CAD build for the part. Positions are in the model's coordinates, mm. A direction names the side the tool comes from. Coordinates: 2 decimals unless noted, no trailing zeros. Order: outer loops, then holes, each group sorted by start corner. A loop starts at its lowest first (then second) coordinate and runs counter-clockwise, first axis right, second up. Notation, with made-up numbers: (78, -15) - (119, -15) arc R12 ccw to (119, 6) - close; hole circle Ø4 at (34, -37). An arc over 180 degrees is marked (long way). Return JSON: item names as keys, results as strings.
from build123d import *


with BuildPart() as f1:
    # F0 (on Right) → F1 (revolve)
    with BuildSketch(Plane.YZ):
        with BuildLine():
            Line((-12.7, 15.875), (-12.7, 16.594964))
            Line((-12.7, 16.594964), (-1.207143, 19.037846))
            ThreePointArc((-1.207143, 19.037846), (-0.33963, 19.569458), (0, 20.528543))
            Line((0, 20.528543), (0, 37.338))
            ThreePointArc((0, 37.338), (-0.223185, 37.876815), (-0.762, 38.1))
            Line((-0.762, 38.1), (-37.338, 38.1))
            ThreePointArc((-37.338, 38.1), (-37.876815, 37.876815), (-38.1, 37.338))
            Line((-38.1, 37.338), (-38.1, 0))
            Line((-38.1, 0), (-19.05, 0))
            Line((-19.05, 0), (-19.05, 15.875))
            Line((-19.05, 15.875), (-12.7, 15.875))
        make_face()
    revolve(axis=Axis((0, -28.575, 0), (0, 1, 0)))


solid = f1.part
Item 1: Band-saw the part on C-C, the plane y = -5.5. List the corners of the cut face in (x, z).
Findings below:
{"outline": "circle Ø76.2 at (0, 0); hole circle Ø36.25 at (0, 0)"}
Item 2: Band-saw the part on B-B, the plane x = 0. List the corners of the cut face in (y, z) (3 decimals), then the cut area to 3 significant figures.
Findings below:
{"outline": "(-38.1, -37.338) arc R0.762 ccw to (-37.338, -38.1) - (-0.762, -38.1) arc R0.762 ccw to (0, -37.338) - (0, -20.529) arc R1.524 ccw to (-1.207, -19.038) - (-12.7, -16.595) - (-12.7, -15.875) - (-19.05, -15.875) - (-19.05, 15.875) - (-12.7, 15.875) - (-12.7, 16.595) - (-1.207, 19.038) arc R1.524 ccw to (0, 20.529) - (0, 37.338) arc R0.762 ccw to (-0.762, 38.1) - (-37.338, 38.1) arc R0.762 ccw to (-38.1, 37.338) - close", "area": "2,240 mm²"}
Item 3: Mould opens along X. For faces 3 (the cylindrical face through (-23.183, -19.306, -30.235)), 4 (the flat face through (-15, -12.7, -6)), 5 (the flat face through (-16, 0, -16)), 6 (the cylindrical face through (-15.497, -15.831, -3.441)) say: released by +X, released by -X, zero draft, split by the parting line, or undercut.
Findings below:
{"face 3": "split by the parting line", "face 4": "undercut", "face 5": "zero draft", "face 6": "undercut"}
Item 4: Wall check: L1, parallel to X at y = -17.25, z = 0 (3 decimals); L2, parallel to Z at x = 33, y = -34; L3, parallel to Y at x = 4, z = 11. Give the ranges that are in metal, low to high. Write a range as [from, to].
Findings below:
{"L1": "x = [-38.1, -15.875], [15.875, 38.1]", "L2": "z = [-19.04, 19.04]", "L3": "y = [-38.1, -19.05]"}
Item 5: Band-saw the part on D-D, the plane y = -24. List the corners of the cut face in (x, z).
Findings below:
{"outline": "circle Ø76.2 at (0, 0)"}
Item 6: Band-saw the part on A-A, the plane z = 0. List the corners of the cut face in (x, y) (3 decimals).
Findings below:
{"outline": "(-38.1, -37.338) arc R0.762 ccw to (-37.338, -38.1) - (37.338, -38.1) arc R0.762 ccw to (38.1, -37.338) - (38.1, -0.762) arc R0.762 ccw to (37.338, 0) - (20.529, 0) arc R1.524 ccw to (19.038, -1.207) - (16.595, -12.7) - (15.875, -12.7) - (15.875, -19.05) - (-15.875, -19.05) - (-15.875, -12.7) - (-16.595, -12.7) - (-19.038, -1.207) arc R1.524 ccw to (-20.529, 0) - (-37.338, 0) arc R0.762 ccw to (-38.1, -0.762) - close"}
Item 7: Which spindle directions (+Z, -Z, +X, -X, +Y, -Y) get a long thin tool onto all of the face, cutting with end or side? Do faces 1 (the flat face through (0, -19.05, 0)), 2 (the flat face through (1, -38.1, -1)). Say none if no direction does.
Findings below:
{"face 1": "+Y", "face 2": "+Z, -Z, +X, -X, -Y"}
Item 8: Drop flat-ended pins along their axis: P1, Ø3, axis at x = 25, y = -4.5, coming from the -Z side; P2, Ø1, axis at x = 13.5, y = -17.5, coming from the -Z side; P3, Ø8, axis at y = -32.5, z = -26, coming from the +X side. Give the stop position or say it passes through.
Findings below:
{"P1": "stops at z = -29.99", "P2": "stops at z = -35.81", "P3": "stops at x = 31.11"}
